Autodesk Fusion 360 part; units mm, degrees
sketch "スケッチ1" plane through (0, 0, 0) normal (0, 0, 1) x (1, 0, 0)
  line L0 (0, 0) -> (-70, 0)
  line L1 (-70, 0) -> (-70, -6)
  line L2 (-70, -6) -> (0, -6)
  line L3 (0, -6) -> (0, 0)
extrude "押し出し1" add sketch "スケッチ1" along normal blind 20
sketch "スケッチ2" plane through (0, -6, 0) normal (0, -1, 0) x (1, 0, 0)
  line L0 (-70, 0) -> (0, 0)
  line L1 (0, 0) -> (0, 20)
  line L2 (0, 20) -> (-70, 20)
  line L3 (-70, 20) -> (-70, 0)
  circle A0 centre (-60, 10) radius 2.05
extrude "押し出し2" cut sketch "スケッチ2" against normal blind 6 contours A0
sketch "スケッチ3" plane through (0, 0, 0) normal (1, 0, 0) x (0, 1, 0)
  line L0 (-6, 0) -> (0, 0)
  line L1 (0, 0) -> (0, 20)
  line L2 (0, 20) -> (-6, 20)
  line L3 (-6, 20) -> (-6, 0)
  circle A0 centre (-3, 5) radius 1.5
  circle A1 centre (-3, 15) radius 1.5
extrude "押し出し3" cut sketch "スケッチ3" against normal blind 6 contours A0 | A1
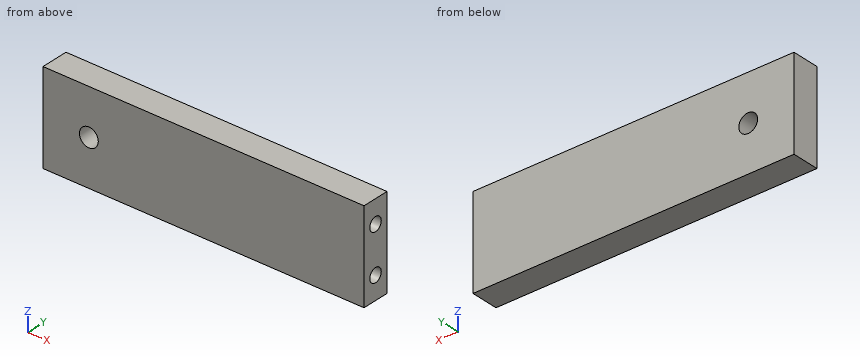
Design review of the part built by this model. Coordinates are the model's own, in mm. Round coordinates to 2 decimals unless told otherwise and drop trailing zeros. Write each loop counter-clockwise with the first axis right and the second up, starting at its lowest first coordinate (ties: lowest second). Pieces come first, ordered by that corner, then holes. Notation, with made-up numbers: M -6.75,39 L 20.25,39 A28 ccw 20.25,73 Z; hole C -10.5,78.25 d6. An arc over 180 degrees is marked long. One line per item, written item: value. Start each with the question number.
1. To check wall thickness, follow probe 1 along Z at (x, y) = (-3.7, -3); probe 2 along Z at (x, y) = (-60, -4.75); probe 3 along X at (y, z) = (-3.95, 4). State the ranges of each line that lie inside material, in increasing order. Write a range as from..to.
2. Clearance check with flat-ended pins moving along their axes: P1, Ø4, axis at x = -26, z = 5.5, coming from the +Y side; P2, Ø1.5, axis at y = -3.5, z = 15, coming from the +X side; P3, Ø2.5, axis at x = -60, z = 10, coming from the +Y side. State where each tip first meets the part, or that it passes through.
3. Take a section at B-B on x = -60. State the section outline as (y, z) points.
4. Take a section at A-A on y = -3. State the section outline as (x, z) points, then the cut area to 3 significant figures.
5. Take a section at C-C on z = 10. State the section outline as (x, y) points, then the cut area to 3 significant figures.
6. Take a section at D-D on z = 15. State the section outline as (x, y) points, then the cut area to 3 significant figures.
Computed:
1. probe 1: z = 0..3.5, 6.5..13.5, 16.5..20
1. probe 2: z = 0..7.95, 12.05..20
1. probe 3: x = -70..-6
2. P1: stops at y = 0
2. P2: stops at x = -6
2. P3: passes through
3. outline: M -6,0 L 0,0 L 0,7.95 L -6,7.95 Z; M -6,12.05 L 0,12.05 L 0,20 L -6,20 Z
4. outline: M -70,0 L 0,0 L 0,3.5 L -6,3.5 L -6,6.5 L 0,6.5 L 0,13.5 L -6,13.5 L -6,16.5 L 0,16.5 L 0,20 L -70,20 Z; hole C -60,10 d4.1
4. area: 1,350 mm²
5. outline: M -70,-6 L -62.05,-6 L -62.05,0 L -70,0 Z; M -57.95,-6 L 0,-6 L 0,0 L -57.95,0 Z
5. area: 395 mm²
6. outline: M -70,-6 L 0,-6 L 0,-4.5 L -6,-4.5 L -6,-1.5 L 0,-1.5 L 0,0 L -70,0 Z
6. area: 402 mm²
